Model file for the job. Use its own axes, mm. A direction names the side the tool comes from. Round coordinates to 2 decimals unless told otherwise and drop trailing zeros. Loops run counter-clockwise (first coordinate to the right, second up) from the corner with the lowest first, then second, coordinate; pieces in that order, holes last. Notation, with made-up numbers: M -38,53.5 L -27,53.5 A19 cw -27,89.5 Z; hole C 81.25,86.5 d1. An arc over 180 degrees is marked long. Use a Markdown table: item, result. Add a question column.
Item 1: Wall check: L1, parallel to Z at x = -302, y = 7; L2, parallel to Z at x = -254, y = 6; L3, parallel to Y at x = -325.5, z = -20. Give the ranges that are in metal, low to high. Write a range as from..to.
Item 2: Saw through at B-B on y = 69. Write the cut outline in (x, z), then the cut area to 3 significant figures.
Item 3: Saw through at A-A on z = 1. Write the cut outline in (x, y).
Item 4: Two-plate mould, pull along X, no slides. Class faces 1 (the flat face through (-258, 31, 175)), 2 (the flat face through (-203, 8, -150)), 3 (the flat face through (-235, 84, 167)): +X half, -X half, draft (parallel to the pull), parting line (faces both ways), or undercut.
Item 5: Saw through at C-C on x = -101. Write the cut outline in (y, z).
Item 6: Pin check, flat tips, straight feed: P1, Ø5.5, axis at x = -302, z = 155, coming from the +Y side; P2, Ø1, axis at x = -324.5, z = -153.5, coming from the -Y side; P3, Ø7.5, axis at x = -397, z = -29, coming from the +Y side. Stop position of each tip, or through.
Item 7: Tool access for faces 4 (the flat face through (-257, 31, -175)), 5 (the flat face through (-113, 5, -160)), 6 (the flat face through (-371, 15, -37.5)): list every direction of +Z, -Z, +X, -X, +Y, -Y with a clear straight run to the whole face (end or side of a thin tool).
Autodesk Inventor part; units mm, degrees
ref_plane "YZ Plane" through (0, 0, 0) normal (1, 0, 0) x (0, 1, 0)
ref_plane "XZ Plane" through (0, 0, 0) normal (0, 1, 0) x (-1, 0, 0)
ref_plane "XY Plane" through (0, 0, 0) normal (0, 0, 1) x (1, 0, 0)
sketch "Sketch1" plane through (0, 0, 0) normal (0, 1, 0) x (-1, 0, 0)
  line L0 (400, 160) -> (0, 160)
  line L1 (0, 160) -> (0, 150)
  line L2 (0, 150) -> (400, 150)
  line L3 (400, 150) -> (400, 160)
  line L4 (400, -150) -> (0, -150)
  line L5 (0, -150) -> (0, -160)
  line L6 (0, -160) -> (400, -160)
  line L7 (400, -160) -> (400, -150)
  line L8 (0, 150) -> (0, 0) construction
  line L9 (0, 0) -> (200, 0) construction
  circle A0 centre (350, 155) radius 3.5
  circle A1 centre (350, -155) radius 3.5
  circle A2 centre (338, 155) radius 3.5
  circle A3 centre (338, -155) radius 3.5
  circle A4 centre (326, 155) radius 3.5
  circle A5 centre (326, -155) radius 3.5
  circle A6 centre (314, 155) radius 3.5
  circle A7 centre (314, -155) radius 3.5
  circle A8 centre (302, 155) radius 3.5
  circle A9 centre (302, -155) radius 3.5
  circle A10 centre (290, 155) radius 3.5
  circle A11 centre (290, -155) radius 3.5
  circle A12 centre (278, 155) radius 3.5
  circle A13 centre (278, -155) radius 3.5
  circle A14 centre (266, 155) radius 3.5
  circle A15 centre (266, -155) radius 3.5
  circle A16 centre (254, 155) radius 3.5
  circle A17 centre (254, -155) radius 3.5
  circle A18 centre (242, 155) radius 3.5
  circle A19 centre (242, -155) radius 3.5
  circle A20 centre (230, 155) radius 3.5
  circle A21 centre (230, -155) radius 3.5
  circle A22 centre (218, 155) radius 3.5
  circle A23 centre (218, -155) radius 3.5
  circle A24 centre (206, 155) radius 3.5
  circle A25 centre (206, -155) radius 3.5
  circle A26 centre (194, 155) radius 3.5
  circle A27 centre (194, -155) radius 3.5
  circle A28 centre (182, 155) radius 3.5
  circle A29 centre (182, -155) radius 3.5
  circle A30 centre (10, 155) radius 3.5
  circle A31 centre (10, -155) radius 3.5
  point P0 (400, 155)
  point P1 (400, -155)
  point P2 (0, -155)
  point P3 (0, 155)
  dimension "d0" = 10
  dimension "d1" = 400
  dimension "d2" = 300
  dimension "d3" = 150
  dimension "d4" = 200
  dimension "d5" = 50
  dimension "d6" = 7
  dimension "d7" = 7
  dimension "d8" = 50
  dimension "d11" = 12
  dimension "d16" = 7
  dimension "d17" = 10
  dimension "d18" = 10
  dimension "d19" = 7
extrude "Extrusion1" add sketch "Sketch1" along normal blind 10
sketch "Sketch2" plane through (0, 10, 0) normal (0, 1, 0) x (1, 0, 0)
  line L0 (-325, -160) -> (-225, -160)
  line L1 (-225, -160) -> (-225, 160)
  line L2 (-225, 160) -> (-325, 160)
  line L3 (-325, 160) -> (-325, -160)
  line L4 (0, 160) -> (-400, 160)
  line L5 (-400, -160) -> (0, -160)
  line L6 (0, -150) -> (-400, -150)
  line L7 (-400, 150) -> (0, 150)
  line L8 (-315, -150) -> (-235, -150)
  line L9 (-235, -150) -> (-235, 150)
  line L10 (-235, 150) -> (-315, 150)
  line L11 (-315, 150) -> (-315, -150)
  line L12 (-325, -90) -> (-415, -90)
  line L13 (-415, -90) -> (-415, 90)
  line L14 (-415, 90) -> (-325, 90)
  line L15 (-325, 90) -> (-325, -90)
  line L16 (-403, -67.5) -> (-338, -67.5)
  line L17 (-338, -67.5) -> (-338, -37.5)
  line L18 (-338, -37.5) -> (-403, -37.5)
  line L19 (-403, -37.5) -> (-403, -67.5)
  line L20 (-403, -15) -> (-338, -15)
  line L21 (-338, -15) -> (-338, 15)
  line L22 (-338, 15) -> (-403, 15)
  line L23 (-403, 15) -> (-403, -15)
  line L24 (-403, 37.5) -> (-338, 37.5)
  line L25 (-338, 37.5) -> (-338, 67.5)
  line L26 (-338, 67.5) -> (-403, 67.5)
  line L27 (-403, 67.5) -> (-403, 37.5)
  circle A0 centre (-320, -155) radius 3.5
  line L28 (0, -160) -> (0, -150)
  circle A1 centre (-320, 155) radius 3.5
  line L29 (-400, 160) -> (-400, 150)
  circle A2 centre (-230, -155) radius 3.5
  circle A3 centre (-230, 155) radius 3.5
  point P0 (0, 0)
  point P1 (-325, 0)
  point P2 (0, -155)
  point P3 (-400, 155)
  dimension "d22" = 0
  dimension "d23" = 0
  dimension "d25" = 10
  dimension "d26" = 10
  dimension "d27" = 80
  dimension "d28" = 225
  dimension "d31" = 180
  dimension "d33" = 60
  dimension "d34" = 90
  dimension "d35" = 30
  dimension "d36" = 30
  dimension "d37" = 30
  dimension "d38" = 65
  dimension "d41" = 12
  dimension "d42" = 22.5
  dimension "d43" = 22.5
  dimension "d44" = 22.5
  dimension "d48" = 5
  dimension "d49" = 7
  dimension "d50" = 5
  dimension "d51" = 7
  dimension "d54" = 90
extrude "Extrusion3" add sketch "Sketch2" along normal blind 10 contours L3 L6 L1 L0 | L3 L7 L11 L6 | L6 L9 L7 L1 | L12 L13 L14 L3 | L7 L3 L2 L1
sketch "Sketch3" plane through (0, 20, 0) normal (0, 1, 0) x (1, 0, 0)
  line L0 (-415, 90) -> (-415, -90)
  line L1 (-415, -33.5) -> (-385, -33.5)
  line L2 (-385, -33.5) -> (-385, -18.5)
  line L3 (-385, -18.5) -> (-415, -18.5)
  line L4 (-415, -18.5) -> (-415, -33.5)
  line L5 (-415, 19) -> (-385, 19)
  line L6 (-385, 19) -> (-385, 34)
  line L7 (-385, 34) -> (-415, 34)
  line L8 (-415, 34) -> (-415, 19)
  line L9 (-403, 15) -> (-338, 15)
  line L10 (-403, -37.5) -> (-338, -37.5)
  point P0 (0, 0)
  dimension "d61" = 0
  dimension "d62" = 30
  dimension "d63" = 15
  dimension "d64" = 15
  dimension "d65" = 4
  dimension "d66" = 4
extrude "Extrusion4" cut sketch "Sketch3" against normal blind 5
sketch "Sketch4" plane through (-400, 0, 160) normal (0, 0, 1) x (1, 0, 0)
  line L0 (100, 0) -> (170, 0)
  line L1 (170, 0) -> (170, 110)
  line L2 (170, 110) -> (165, 110)
  line L3 (165, 110) -> (165, 57.5278)
  line L4 (100, 0) -> (100, 20)
  line L5 (75, 20) -> (175, 20)
  line L6 (165, 57.5278) -> (100, 20)
  line L7 (175, 10) -> (175, 20)
  point P0 (400, 0)
  dimension "d69" = 120
  dimension "d70" = 5
  dimension "d71" = 110
  dimension "d72" = 70
  dimension "d73" = 20
  dimension "d74" = 5
extrude "Extrusion5" add sketch "Sketch4" along normal blind 15
sketch "Sketch5" plane through (0, 0, -160) normal (0, 0, -1) x (-1, 0, 0)
  line L0 (300, 0) -> (230, 0)
  line L1 (300, 0) -> (230, 0)
  line L2 (230, 0) -> (230, 110)
  line L3 (230, 110) -> (235, 110)
  line L4 (235, 110) -> (235, 57.5278)
  line L5 (325, 20) -> (225, 20)
  line L6 (235, 57.5278) -> (300, 20)
  line L7 (300, 20) -> (300, 0)
  point P0 (0, 0)
  point P1 (230, 20)
  dimension "d83" = 110
  dimension "d84" = 120
  dimension "d85" = 5
extrude "Extrusion6" add sketch "Sketch5" along normal blind 15
properties part number "Pedal Box Mount V1"
Entries:
| question | item | result |
|---|---|---|
| 1 | L1 | -160..-158.5, -151.5..-150, 150..151.5, 158.5..160 |
| 1 | L2 | -175..-158.5, -151.5..-150, 150..151.5, 158.5..175 |
| 1 | L3 | 10..20 |
| 2 | outline | M -235,-175 L -230,-175 L -230,-160 L -235,-160 Z; M -235,160 L -230,160 L -230,175 L -235,175 Z |
| 2 | area | 150 mm2 |
| 3 | outline | M -415,10 L -403,10 L -403,20 L -415,20 Z; M -338,10 L -315,10 L -315,20 L -338,20 Z; M -235,10 L -225,10 L -225,20 L -235,20 Z |
| 4 | face 1 | draft |
| 4 | face 2 | undercut |
| 4 | face 3 | -X half |
| 5 | outline | M 0,-160 L 10,-160 L 10,-150 L 0,-150 Z; M 0,150 L 10,150 L 10,160 L 0,160 Z |
| 6 | P1 | y = 20 |
| 6 | P2 | y = 10 |
| 6 | P3 | y = 15 |
| 7 | face 4 | -Z, +X, -X, +Y, -Y |
| 7 | face 5 | -Z, +X, +Y, -Y |
| 7 | face 6 | +Y, -Y |
